Geometry check sheet. Reference: the model listing, model coordinates, mm. A direction names the side the tool comes from. Round coordinates to 2 decimals unless told otherwise and drop trailing zeros. Loops run counter-clockwise (first coordinate to the right, second up) from the corner with the lowest first, then second, coordinate; pieces in that order, holes last. Notation, with made-up numbers: (35.5, -23) - (59.5, -23) arc R24 cw to (59.5, 15) - close; hole circle Ø5 at (-12.5, -8.75). An arc over 180 degrees is marked (long way). Answer as CSV lines item,"result". Start each with the question number.
1) Depth check by flat-ended pin: P1, Ø4, axis at y = -121.5, z = -53, coming from the -X side; P2, Ø14.5, axis at y = 133.25, z = -62.5, coming from the -X side; P3, Ø18.5, axis at y = 25, z = 125, coming from the -X side; P4, Ø6, axis at y = -85, z = -95.5, coming from the +X side. Enter the tip coordinate at first touch or a pass-through.
2) Thickness scan on line 1 along Z through (x, y) = (-85.25, 25); line 2 along Y through (x, z) = (-11, 0); line 3 along X through (y, z) = (144, -51.5). Record the ranges inside material, lowest first.
3) Cross-section at B-B on z = 0. State how many separate pieces and enclosed holes the cut face has, and give its area (3 significant figures).
4) Cross-section at A-A on x = -102.5. Record the boundary of the cut face in (y, z).
5) Access from +Z, -Z, +X, -X, +Y, -Y to the whole of each face (thin tool, end or side, straight path). Record for faces 1 (the cylindrical face through (-87.077, 89.234, 100.443)), 2 (the conical face through (-132.383, -8.793, 152.178)).
6) Draft check along Y on faces 3 (the cylindrical face through (-87, -92, 0)), 4 (the conical face through (-246.78, 121.48, -185.49)). Enter one of: released by +Y, released by -Y, zero draft, split by the parting line, or undercut.
Autodesk Fusion 360 part; units mm, degrees
sketch "Sketch1" plane through (0, 0, 0) normal (0, 0, 1) x (1, 0, 0)
  line L0 (-86.9849, 25) -> (-86.9849, 125)
  line L1 (-86.9849, 125) -> (-80.4008, 125)
  line L2 (-80.4008, 125) -> (-80.4008, 175)
  line L3 (-80.4008, 175) -> (-40.4008, 175)
  line L4 (-40.4008, 175) -> (-26.2586, 189.1421)
  line L5 (-26.2586, 189.1421) -> (33.7414, 189.1421)
  line L6 (33.7414, 189.1421) -> (71.4286, 219.1421)
  line L7 (71.4286, 219.1421) -> (73.1213, 234.0463)
  line L8 (-85.2557, 180) -> (-42.4718, 180)
  line L9 (-42.4718, 180) -> (-28.3297, 194.1421)
  line L10 (-28.3297, 194.1421) -> (31.9943, 194.1421)
  line L11 (31.9943, 194.1421) -> (66.6943, 221.7642)
  line L12 (66.6943, 221.7642) -> (68.1532, 234.6105)
  line L13 (68.1532, 234.6105) -> (73.1213, 234.0463)
  line L14 (-93.5691, 125) -> (-93.5691, 175)
  line L15 (-242.1231, 234.6105) -> (-247.0911, 234.0463)
  line L16 (-205.9641, 194.1421) -> (-240.6641, 221.7642)
  line L17 (-240.6641, 221.7642) -> (-242.1231, 234.6105)
  line L18 (-145.6402, 194.1421) -> (-205.9641, 194.1421)
  line L19 (-86.9849, 125) -> (-93.5691, 125)
  line L20 (-147.7112, 189.1421) -> (-207.7112, 189.1421)
  line L21 (-93.5691, 175) -> (-133.5691, 175)
  line L22 (-245.3985, 219.1421) -> (-247.0911, 234.0463)
  line L23 (-88.7142, 180) -> (-131.498, 180)
  line L24 (-86.9849, 25) -> (-86.9849, 125)
  line L25 (-131.498, 180) -> (-145.6402, 194.1421)
  line L26 (-133.5691, 175) -> (-147.7112, 189.1421)
  line L27 (-207.7112, 189.1421) -> (-245.3985, 219.1421)
  line L28 (-85.2557, 180) -> (-88.7142, 180)
  line L29 (-86.9849, 25) -> (-270, 25)
  point P0 (-173.9699, 0)
  dimension "d1" = 100
  dimension "d2" = 40
  dimension "d3" = 20
  dimension "d4" = 135
  dimension "d5" = 60
  dimension "d6" = 30
  dimension "d7" = 15
  dimension "d8" = 135
  dimension "d10" = -5
  dimension "d11" = 50
revolve "Revolve1" add sketch "Sketch1" angle 360 about axis through (-86.9849, 25, 0) along (-1, 0, 0)
sketch "Sketch2" plane through (-93.5691, 0, 0) normal (-1, 0, 0) x (0, -1, 0)
  circle A0 centre (-25, 0) radius 100
  circle A1 centre (-25, 0) radius 150
  line L0 (-25, 0) -> (-25, -125)
  circle A2 centre (-25, -125) radius 8
  circle A3 centre (37.5, -108.2532) radius 8
  circle A4 centre (83.2532, -62.5) radius 8
  circle A5 centre (100, 0) radius 8
  circle A6 centre (83.2532, 62.5) radius 8
  circle A7 centre (37.5, 108.2532) radius 8
  circle A8 centre (-25, 125) radius 8
  circle A9 centre (-87.5, 108.2532) radius 8
  circle A10 centre (-133.2532, 62.5) radius 8
  circle A11 centre (-150, 0) radius 8
  circle A12 centre (-133.2532, -62.5) radius 8
  circle A13 centre (-87.5, -108.2532) radius 8
  dimension "d13" = 16
  dimension "d15" = 360
extrude "Extrude1" cut sketch "Sketch2" against normal blind 200 contours A2 | A3 | A4 | A5 | A6 | A7 | A8 | A9 | A10 | A11 | A12 | A13
Answer block:
1,P1,"stops at x = -141.36"
1,P2,"passes through"
1,P3,"stops at x = -93.57"
1,P4,"stops at x = -80.4"
2,line 1,"z = -155 to -133, -117 to -100, 100 to 117, 133 to 155"
2,line 2,"y = -144.14 to -139.14, 189.14 to 194.14"
2,line 3,"x = -93.57 to -80.4"
3,separate pieces,"4"
3,enclosed holes,"0"
3,area,"4,610 mm^2"
4,outline,"circle Ø310 at (25, 0); hole circle Ø300 at (25, 0)"
5,face 1,"+X, -X"
5,face 2,"none"
6,face 3,"undercut"
6,face 4,"split by the parting line"
